Model file for the job. Use its own axes, mm. A direction names the side the tool comes from. Round coordinates to 2 decimals unless told otherwise and drop trailing zeros. Order: outer loops, then holes, each group sorted by start corner. A loop starts at its lowest first (then second) coordinate and runs counter-clockwise, first axis right, second up. Notation, with made-up numbers: (78, 6.5) -> (135, 6.5) arc R19 ccw to (135, 16.5) -> close; hole circle Ø6 at (8.5, -20). An arc over 180 degrees is marked (long way). Put each result on its own line as item: value. Start each with the question number.
Q1. 3-axis set-ups, long thin cutter, end or side, ignore diameter. For faces 1 (the face through (88, 12, 2)), 2 (the face through (59.41, 0.53, -11.99)), 3 (the face through (13.521, -7.91, -10.316)), 4 (the face through (30, 12, 2)), 5 (the face through (68, -20.2, 0.4)): which of +Z, -Z, +X, -X, +Y, -Y reach the whole face in a straight line?
Q2. Pull direction Y, two halves, no side cores. Call faces 6 (the face through (85, 16.4, -1.4)), 7 (the face through (1.5, -16.3, -0.3)), 8 (the face through (26.06, -15.62, -3.47)), 9 (the face through (76.381, -19.524, -4.336)): released by +Y, released by -Y, zero draft, split by the parting line, or undercut.
Q3. Cut at B-B, the plane x = 37. List the corners of the cut face in (y, z), and give its area (3 significant figures).
Q4. Cut at A-A, the plane x = 8.5. List the corners of the cut face in (y, z), and give its area (3 significant figures).
Q5. Probe L1, parallel to X at y = -7, z = 13.5; L2, parallel to X at y = -17.5, z = -2.5; L3, parallel to Y at x = 59.5, z = 0. List the from-to ranges inside material, lowest first.
Q6. Flat gauge pins, fed straight in: P1, Ø3, axis at x = 53, z = -11, coming from the +Y side; P2, Ø15.5, axis at y = 0, z = 0, coming from the +X side; P3, Ø1.5, axis at x = 65, y = 9.5, coming from the -Z side; P4, Ø6, axis at x = 29.5, y = 16, coming from the -Z side. Where does each tip first touch, or does it go through?
from build123d import *


with BuildPart() as f1:
    # F0 (on Front) → F1 (revolve)
    with BuildSketch(Plane.XZ):
        with BuildLine():
            ThreePointArc((6, 31), (1.757359, 29.242641), (0, 25))
            Line((0, 25), (1.5, 25))
            Line((1.5, 25), (1.5, 16))
            Line((1.5, 16), (12, 16))
            Line((12, 16), (12, 13))
            Line((12, 13), (15, 13))
            Line((15, 13), (15, 20.5))
            Line((15, 20.5), (22, 20.5))
            Line((22, 20.5), (22, 16))
            Line((22, 16), (30, 16))
            Line((30, 16), (30, 12))
            Line((30, 12), (88, 12))
            Line((88, 12), (88, 16.124999))
            Line((88, 16.124999), (85, 16.124999))
            Line((85, 16.124999), (85, 20))
            Line((85, 20), (68, 20))
            Line((68, 20), (68, 31))
            Line((68, 31), (56, 31))
            ThreePointArc((56, 31), (50, 25), (44, 31))
            Line((44, 31), (6, 31))
        make_face()
    revolve(axis=Axis((44, 0, 0), (-1, 0, 0)))


solid = f1.part
Ans:
1. face 1: +Z, -Z, +X, +Y, -Y
1. face 2: +X, -X
1. face 3: -X
1. face 4: none
1. face 5: +X
2. face 6: zero draft
2. face 7: undercut
2. face 8: undercut
2. face 9: split by the parting line
3. outline: circle Ø62 at (0, 0); hole circle Ø24 at (0, 0)
3. area: 2,570 mm^2
4. outline: circle Ø62 at (0, 0); hole circle Ø32 at (0, 0)
4. area: 2,210 mm^2
5. L1: x = 12 to 15, 30 to 88
5. L2: x = 1.5 to 15, 22 to 85
5. L3: y = -31 to -12, 12 to 31
6. P1: stops at y = 24.81
6. P2: passes through
6. P3: stops at z = -29.74
6. P4: stops at z = -28.14
